from build123d import *

# Parameters (mm, degrees)
SKETCH1_R                = 3.875
BOSS_EXTRUDE1_DEPTH      = 9
BOSS_EXTRUDE1_DEPTH_BACK = 4
SKETCH2_R                = 5.4
BOSS_EXTRUDE2_DEPTH      = 9
SKETCH7_R                = 10
BOSS_EXTRUDE4_DEPTH      = 8
CUT_EXTRUDE2_START       = -9
SKETCH3_R                = 1.425
CUT_EXTRUDE2_DEPTH       = 10
SKETCH6_R                = 2.65
CUT_EXTRUDE3_DEPTH       = 6
CIRPATTERN1_COUNT        = 2
SKETCH8_R                = 2.25
CUT_EXTRUDE4_DEPTH       = 1
CUT_EXTRUDE4_DEPTH_BACK  = 14


with BuildPart() as part:
    # Sketch1 → Boss-Extrude1 (new body, two sides)
    with BuildSketch(Plane(origin=(0, 0, 0), x_dir=(1, 0, 0), z_dir=(0, 1, 0))) as boss_extrude1_sk:
        Circle(SKETCH1_R)
    extrude(amount=BOSS_EXTRUDE1_DEPTH)
    extrude(boss_extrude1_sk.sketch, amount=-BOSS_EXTRUDE1_DEPTH_BACK)

    # Sketch2 → Boss-Extrude2 (add)
    with BuildSketch(Plane(origin=(0, 0, 0), x_dir=(1, 0, 0), z_dir=(0, 1, 0))):
        Circle(SKETCH2_R)
    extrude(amount=BOSS_EXTRUDE2_DEPTH)

    # Sketch7 → Boss-Extrude4 (add)
    with BuildSketch(Plane(origin=(0, 9, 0), x_dir=(1, 0, 0), z_dir=(0, 1, 0))):
        Circle(SKETCH7_R)
    extrude(amount=-BOSS_EXTRUDE4_DEPTH)

    # Sketch3 → Cut-Extrude2 (cut)
    with BuildSketch(Plane(origin=(0, 9, 0), x_dir=(1, 0, 0), z_dir=(0, 1, 0)).offset(CUT_EXTRUDE2_START)):
        with Locations((-7.75, 0)):
            Circle(SKETCH3_R)
    cut_extrude2 = extrude(amount=CUT_EXTRUDE2_DEPTH, mode=Mode.SUBTRACT)

    # Sketch6 → Cut-Extrude3 (cut)
    with BuildSketch(Plane(origin=(0, 9, 0), x_dir=(1, 0, 0), z_dir=(0, 1, 0))):
        with Locations((-7.75, 0)):
            Circle(SKETCH6_R)
    cut_extrude3 = extrude(amount=-CUT_EXTRUDE3_DEPTH, mode=Mode.SUBTRACT)

    # CirPattern1: Cut-Extrude2, Cut-Extrude3 ×2 about axis
    cirpattern1_axis = Axis((0, 0, 0), (0, 1, 0))
    for i in range(1, CIRPATTERN1_COUNT):
        add(cut_extrude2.rotate(cirpattern1_axis, i * 360 / CIRPATTERN1_COUNT), mode=Mode.SUBTRACT)
        add(cut_extrude3.rotate(cirpattern1_axis, i * 360 / CIRPATTERN1_COUNT), mode=Mode.SUBTRACT)

    # Sketch8 → Cut-Extrude4 (cut, two sides)
    with BuildSketch(Plane.XZ.offset(4)) as cut_extrude4_sk:
        Circle(SKETCH8_R)
    extrude(amount=CUT_EXTRUDE4_DEPTH, mode=Mode.SUBTRACT)
    extrude(cut_extrude4_sk.sketch, amount=-CUT_EXTRUDE4_DEPTH_BACK, mode=Mode.SUBTRACT)


solid = part.part
The model under review builds one solid part; all positions refer to its coordinate system, in mm. A direction names the side the tool comes from. Round coordinates to 2 decimals unless told otherwise and drop trailing zeros. Loops run counter-clockwise (first coordinate to the right, second up) from the corner with the lowest first, then second, coordinate; pieces in that order, holes last. Notation, with made-up numbers: (76, -16.5) -> (88, -16.5) arc R19 cw to (88, -9.5) -> close; hole circle Ø4 at (19, 67.25). An arc over 180 degrees is marked (long way). Return JSON: item names as keys, results as strings.
(1) For line 1 (Z direction, x = -7.75, y = 1.6) (3 decimals); line 2 (Z direction, x = -7.75, y = 4.3); line 3 (X direction, y = 7.5, z = 2), list the stretches that pass through material, from the lowest coordinate up.
Solved:
{"line 1": "-6.32 to -1.425, 1.425 to 6.32", "line 2": "-6.32 to -2.65, 2.65 to 6.32", "line 3": "-9.8 to -9.49, -6.01 to -1.03, 1.03 to 6.01, 9.49 to 9.8"}
(2) Add section B-B on z = 0. Write out the cut boundary in (x, y) (3 decimals).
Solved:
{"outline": "(-10, 1) -> (-9.175, 1) -> (-9.175, 3) -> (-10, 3) -> close; (-6.325, 1) -> (-5.4, 1) -> (-5.4, 0) -> (-3.875, 0) -> (-3.875, -4) -> (-2.25, -4) -> (-2.25, 9) -> (-5.1, 9) -> (-5.1, 3) -> (-6.325, 3) -> close; (2.25, -4) -> (3.875, -4) -> (3.875, 0) -> (5.4, 0) -> (5.4, 1) -> (6.325, 1) -> (6.325, 3) -> (5.1, 3) -> (5.1, 9) -> (2.25, 9) -> close; (9.175, 1) -> (10, 1) -> (10, 3) -> (9.175, 3) -> close"}
(3) For pin 1 (5 mm diameter, centred on y = 5.5, z = 2.5, fed in from +X); pin 2 (10 mm diameter, centred on x = -6, z = 3, fed in from -Y); pin 3 (2.5 mm diameter, centred on x = 7.75, z = 0, fed in from +Y); pin 4 (1 mm diameter, centred on y = -2, z = 0, fed in from +X) (3 decimals), all flat-tipped, find the tip position at first contact; note any pin that passes through.
Solved:
{"pin 1": "x = 9.87", "pin 2": "y = -4", "pin 3": "through", "pin 4": "x = 3.875"}
(4) The part is to be moulded in two halves that separate along Z. For faces 4 (the flat face through (-1, 0, -4)), 5 (the cylindrical face through (-1.17, 0.49, 5.27)), 6 (the flat face through (-9, 3, 1)), say which applies: released by +Z, released by -Z, zero draft, split by the parting line, or undercut.
Solved:
{"face 4": "zero draft", "face 5": "split by the parting line", "face 6": "undercut"}
(5) For faces 1 (the cylindrical face through (-0.29, 2.41, 2.23)), 2 (the cylindrical face through (-0.504, -1.972, -3.842)), 3 (the flat face through (9, 3, -1)), list the 3-axis set-ups (+Z, -Z, +X, -X, +Y, -Y) from which the entire face can be reached by the end or side of a thin tool; tool diameter is ignored.
Solved:
{"face 1": "+Y, -Y", "face 2": "-Y", "face 3": "+Y"}
(6) Add section D-D on y = 0.25. Write out the cut boundary in (x, z).
Solved:
{"outline": "circle Ø10.8 at (0, 0); hole circle Ø4.5 at (0, 0)"}
(7) Add section A-A on x = 0. Write out the cut boundary in (y, z) (3 decimals).
Solved:
{"outline": "(-4, -3.875) -> (0, -3.875) -> (0, -5.4) -> (1, -5.4) -> (1, -10) -> (9, -10) -> (9, -2.25) -> (-4, -2.25) -> close; (-4, 2.25) -> (9, 2.25) -> (9, 10) -> (1, 10) -> (1, 5.4) -> (0, 5.4) -> (0, 3.875) -> (-4, 3.875) -> close"}
(8) Add section C-C on y = 2. Write out the cut boundary in (x, z) (3 decimals), plus the area to 3 significant figures.
Solved:
{"outline": "circle Ø20 at (0, 0); hole circle Ø2.85 at (-7.75, 0); hole circle Ø4.5 at (0, 0); hole circle Ø2.85 at (7.75, 0)", "area": "285 mm2"}
